Check sheet for the modelled part. Datum: model origin and axes. Units: mm. A direction names the side the tool comes from. Coordinates: 2 decimals unless noted, no trailing zeros. Loops run counter-clockwise (first coordinate to the right, second up) from the corner with the lowest first, then second, coordinate; pieces in that order, holes last. Notation, with made-up numbers: M -21.5,66 L 20.5,66 A26 ccw 20.5,87 Z; hole C 89.5,86 d8. An arc over 180 degrees is marked long. Use CSV: the item, a comma, the result in double quotes. Start each with the question number.
(1) Section check A-A on x = 4. Record the cut outline in (y, z), and give its area (3 significant figures).
(2) Section check D-D on y = -2.5. Record the cut outline in (x, z), and give its area (3 significant figures).
(3) Set-up check for faces 1 (the cylindrical face through (-13.52, -14.13, 1.23)), 2 (the flat face through (2, -8.468, 1)): record each of +Z, -Z, +X, -X, +Y, -Y from which the full face is reachable in a straight line by a thin tool's end or side.
(4) Section check C-C on z = 0.8. Give the number of separate pieces and of enclosed holes in the cut face, and give its area (3 significant figures).
(5) Section check B-B on y = -18.25. Record the cut outline in (x, z).
(6) Go/stop test with flat-tipped pins: pin 1 Ø0.6 at (y, z) = (-8, 1) entering from -X; pin 2 Ø0.8 at (x, z) = (4.5, 1) entering from +Y; pin 3 Ø1 at (y, z) = (-22, 0.5) entering from -X. Record where each tip stops, or that it passes through.
(7) Draft check along X on faces 3 (the flat face through (-6.806, -9.486, 1.232)), 4 (the flat face through (-3.2, -10.9, 2.5)), 5 (the flat face through (-7, -7, 1)), 6 (the cylindrical face through (13.52, -14.16, 1.23)). Enter one of: pulls with the +X half, pulls with the -X half, needs draft (parallel to the pull), parting line crosses it, or undercut.
(8) Scan lines: line 1 (X direction, y = -12.75, z = 2.1); line 2 (Y direction, x = 2.75, z = 0.35); line 3 (Y direction, x = 7.75, z = 0.85). Record each from-to range of solid material in increasing order.
from build123d import *

# Parameters (mm, degrees)
F1_DEPTH = 2.5
F2_R     = 0.85
F3_DEPTH = 12.5


with BuildPart() as f1:
    # F0 (on Top) → F1 (new body)
    with BuildSketch(Plane.XY):
        with BuildLine():
            Line((13.081475452, -13.081475452), (1.0606601718, -1.0606601718))
            ThreePointArc((1.0606601718, -1.0606601718), (0, -0.6213203436), (-1.0606601718, -1.0606601718))
            Line((-1.0606601718, -1.0606601718), (-13.081475452, -13.081475452))
            ThreePointArc((-13.081475452, -13.081475452), (-13.5208152802, -14.1421356237), (-13.081475452, -15.2027957955))
            Line((-13.081475452, -15.2027957955), (-1.0606601718, -27.2236110757))
            ThreePointArc((-1.0606601718, -27.2236110757), (0, -27.6629509039), (1.0606601718, -27.2236110757))
            Line((1.0606601718, -27.2236110757), (13.081475452, -15.2027957955))
            ThreePointArc((13.081475452, -15.2027957955), (13.5208152802, -14.1421356237), (13.081475452, -13.081475452))
        make_face()
        with BuildLine():
            Line((-1.559338312, -7.9764372607), (-2.8852931731, -12.9341195524))
            Line((-2.8852931731, -12.9341195524), (-3.4549546314, -12.9341195524))
            Line((-3.4549546314, -12.9341195524), (-4.4553886592, -9.6148921218))
            add(Edge.make_bspline(
                [(-4.4553886592, -9.6148921218), (-4.5270032425, -9.3935379552), (-4.6148938675, -9.0582514968)],
                knots=[0, 0, 0, 1, 1, 1], degree=2))
            add(Edge.make_bspline(
                [(-4.6148938675, -9.0582514968), (-4.7027844925, -8.7229650385), (-4.7060397009, -8.6546056635)],
                knots=[0, 0, 0, 1, 1, 1], degree=2))
            add(Edge.make_bspline(
                [(-4.7060397009, -8.6546056635), (-4.7809094925, -9.102739344), (-4.9436699092, -9.6344233718)],
                knots=[0, 0, 0, 1, 1, 1], degree=2))
            Line((-4.9436699092, -9.6344233718), (-5.9137219925, -12.9341195524))
            Line((-5.9137219925, -12.9341195524), (-6.4833834509, -12.9341195524))
            Line((-6.4833834509, -12.9341195524), (-7.8028278953, -7.9764372607))
            Line((-7.8028278953, -7.9764372607), (-7.1919337981, -7.9764372607))
            Line((-7.1919337981, -7.9764372607), (-6.4085136592, -11.0385032329))
            add(Edge.make_bspline(
                [(-6.4085136592, -11.0385032329), (-6.2457532425, -11.6830344829), (-6.1708834509, -12.2049528857)],
                knots=[0, 0, 0, 1, 1, 1], degree=2))
            add(Edge.make_bspline(
                [(-6.1708834509, -12.2049528857), (-6.0797376175, -11.5842931635), (-5.8996160898, -10.9907601774)],
                knots=[0, 0, 0, 1, 1, 1], degree=2))
            Line((-5.8996160898, -10.9907601774), (-5.0120292842, -7.9764372607))
            Line((-5.0120292842, -7.9764372607), (-4.401135187, -7.9764372607))
            Line((-4.401135187, -7.9764372607), (-3.4690605342, -11.0178869135))
            add(Edge.make_bspline(
                [(-3.4690605342, -11.0178869135), (-3.3063001175, -11.544145594), (-3.1945379648, -12.2049528857)],
                knots=[0, 0, 0, 1, 1, 1], degree=2))
            add(Edge.make_bspline(
                [(-3.1945379648, -12.2049528857), (-3.1294337981, -11.7231820524), (-2.9503973398, -11.0319928163)],
                knots=[0, 0, 0, 1, 1, 1], degree=2))
            Line((-2.9503973398, -11.0319928163), (-2.1702324092, -7.9764372607))
            Line((-2.1702324092, -7.9764372607), (-1.559338312, -7.9764372607))
        make_face(mode=Mode.SUBTRACT)
        with BuildLine():
            Line((-8.1334756687, -14.8039748892), (-8.1334756687, -13.4802963582))
            Line((-8.1334756687, -13.4802963582), (-0.6236797201, -13.4802963582))
            Line((-0.6236797201, -13.4802963582), (-0.6236797201, -6.9198086858))
            ThreePointArc((-0.6236797201, -6.9198086858), (-0.9032194318, -6.4583786209), (-0.9135835525, -5.9189782686))
            ThreePointArc((-0.9135835525, -5.9189782686), (0.0168397474, -5.0141534426), (0.9868078824, -5.876451129))
            ThreePointArc((0.9868078824, -5.876451129), (0.9900106564, -6.4384308628), (0.6999988109, -6.9198086858))
            Line((0.6999988109, -6.9198086858), (0.6999988109, -13.4802963582))
            Line((0.6999988109, -13.4802963582), (8.1334756687, -13.4802963582))
            ThreePointArc((8.1334756687, -13.4802963582), (8.5949057336, -13.2007566465), (9.134306086, -13.1903925258))
            ThreePointArc((9.134306086, -13.1903925258), (10.0391309119, -14.1208158258), (9.1768332255, -15.0907839607))
            ThreePointArc((9.1768332255, -15.0907839607), (8.6148534917, -15.0939867347), (8.1334756687, -14.8039748892))
            Line((8.1334756687, -14.8039748892), (0.6999988109, -14.8039748892))
            Line((0.6999988109, -14.8039748892), (0.6999988109, -23.1867600232))
            Line((0.6999988109, -23.1867600232), (-0.6236797201, -23.1867600232))
            Line((-0.6236797201, -23.1867600232), (-0.6236797201, -14.8039748892))
            Line((-0.6236797201, -14.8039748892), (-8.1334756687, -14.8039748892))
        make_face(mode=Mode.SUBTRACT)
        Polygon((3.6052975431, -8.467799659), (3.6052975431, -12.9133291729), (3.0291256681, -12.9133291729), (3.0291256681, -8.467799659), (1.459030182, -8.467799659), (1.459030182, -7.9556468812), (5.1753930292, -7.9556468812), (5.1753930292, -8.467799659), align=None, mode=Mode.SUBTRACT)
    extrude(amount=F1_DEPTH)

    # F2 (on Right) → F3 (cut, symmetric)
    with BuildSketch(Plane.YZ):
        with Locations((-2.4908210296, 1.292226194)):
            Circle(F2_R)
    extrude(amount=F3_DEPTH, both=True, mode=Mode.SUBTRACT)


solid = f1.part
Outcome:
1,outline,"M -24.28,0 L -14.8,0 L -14.8,2.5 L -24.28,2.5 Z; M -13.48,0 L -8.47,0 L -8.47,2.5 L -13.48,2.5 Z; M -7.96,0 L -4,0 L -4,2.5 L -7.96,2.5 Z"
1,area,"46.1 mm²"
2,outline,"M -2.5,0 L 2.5,0 L 2.5,0.44 L -2.5,0.44 Z; M -2.5,2.14 L 2.5,2.14 L 2.5,2.5 L -2.5,2.5 Z"
2,area,"4.00 mm²"
3,face 1,"+Z, -Z, -X"
3,face 2,"+Z, -Z"
4,separate pieces,"2"
4,enclosed holes,"3"
4,area,"329 mm²"
5,outline,"M -10.03,0 L -0.62,0 L -0.62,2.5 L -10.03,2.5 Z; M 0.7,0 L 10.03,0 L 10.03,2.5 L 0.7,2.5 Z"
6,pin 1,"stops at x = -8.3"
6,pin 2,"stops at y = -4.1"
6,pin 3,"stops at x = -6.78"
7,face 3,"undercut"
7,face 4,"needs draft"
7,face 5,"pulls with the -X half"
7,face 6,"pulls with the +X half"
8,line 1,"x = -12.75 to -6.53, -5.86 to -3.51, -2.84 to -0.62, 0.7 to 3.03, 3.61 to 12.75"
8,line 2,"y = -25.53 to -14.8, -13.48 to -8.47, -7.96 to -2.75"
8,line 3,"y = -20.53 to -14.8, -13.48 to -7.75"
